```python
from build123d import *

# Parameters (mm, degrees)
F0_R     = 76.2
F0_W     = 60.587234
F0_H     = 3.302
F1_DEPTH = 12.7


with BuildPart() as f1:
    # F0 (on Front) → F1 (new body)
    with BuildSketch(Plane.XZ):
        Circle(F0_R)
        with Locations((37.913617, -11.811)):
            Rectangle(F0_W, F0_H, mode=Mode.SUBTRACT)
        with BuildLine():
            ThreePointArc((0, -6.35), (-6.35, 0), (0, 6.35))
            Line((0, 6.35), (0, 10.16))
            Line((0, 10.16), (7.62, 10.16))
            Line((7.62, 10.16), (7.62, 1.651))
            Line((7.62, 1.651), (68.58, 1.651))
            Line((68.58, 1.651), (68.58, -1.651))
            Line((68.58, -1.651), (7.62, -1.651))
            Line((7.62, -1.651), (7.62, -10.16))
            Line((7.62, -10.16), (0, -10.16))
            Line((0, -10.16), (0, -6.35))
        make_face(mode=Mode.SUBTRACT)
        with Locations((37.913617, 11.811)):
            Rectangle(F0_W, F0_H, mode=Mode.SUBTRACT)
        with BuildLine():
            ThreePointArc((0, 6.35), (4.490128, 4.490128), (6.35, 0))
            Line((6.35, 0), (7.62, 0))
            Line((7.62, 0), (7.62, 1.651))
            Line((7.62, 1.651), (7.62, 10.16))
            Line((7.62, 10.16), (0, 10.16))
            Line((0, 10.16), (0, 6.35))
        make_face()
        with BuildLine():
            Line((7.62, 0), (6.35, 0))
            ThreePointArc((6.35, 0), (4.490128, -4.490128), (0, -6.35))
            Line((0, -6.35), (0, -10.16))
            Line((0, -10.16), (7.62, -10.16))
            Line((7.62, -10.16), (7.62, -1.651))
            Line((7.62, -1.651), (7.62, 0))
        make_face()
        Polygon((7.62, 1.651), (7.62, 0), (7.62, -1.651), (68.58, -1.651), (68.58, 1.651), align=None)
    extrude(amount=F1_DEPTH)


solid = f1.part
```
Part model, mm, in its own coordinate system. A direction names the side the tool comes from. Coordinates: 2 decimals unless noted, no trailing zeros. Order: outer loops, then holes, each group sorted by start corner. A loop starts at its lowest first (then second) coordinate and runs counter-clockwise, first axis right, second up. Notation, with made-up numbers: (-1, 11) -> (27, 11) arc R15 ccw to (27, 27) -> close; hole circle Ø6 at (-26, 88.25). An arc over 180 degrees is marked (long way). Put each result on its own line as item: value. Start each with the question number.
(1) Which spindle directions (+Z, -Z, +X, -X, +Y, -Y) get a long thin tool onto all of the face, cutting with end or side? Do faces 4 (the face through (16, -12.7, 1)), 5 (the face through (68.207, -6, -12)). Say none if no direction does.
(2) Mould opens along Z. For faces 1 (the face through (-60.47, -6.261, -46.367)), 2 (the face through (68.207, -6, 12)), 3 (the face through (16, 0, 1)) say: pulls with the +Z half, pulls with the -Z half, needs draft (parallel to the pull), parting line crosses it, or undercut.
(3) Band-saw the part on A-A (y = -6.5). Give the cut face in (x, z), then the cut area to 3 significant figures.
(4) Pin check, flat tips, straight feed: pin 1 Ø1.7 at (y, z) = (-6, -12) entering from +X; pin 2 Ø4 at (x, y) = (52, -6.5) entering from -Z; pin 3 Ø3 at (x, y) = (2, -11) entering from -Z; pin 4 Ø1 at (x, z) = (3, -36.5) entering from +Y. Stop position of each tip, or through.
(5) Band-saw the part on C-C (z = -54). Give the cut face in (x, y).
(6) Band-saw the part on D-D (x = -47.5). Give the cut face in (y, z), then the cut area to 3 significant figures.
(7) Band-saw the part on B-B (x = 62.5). Give the cut face in (y, z), then the cut area to 3 significant figures.
(8) Probe line 1 along Z through (x, y) = (61, -11.5); line 2 along Z through (x, y) = (36, -1); line 3 along X through (y, z) = (-5, 2). List the from-to ranges inside material, lowest first. Write a range as [from, to].
Determined:
1. face 4: +Z, -Z, +X, -X, -Y
1. face 5: +Y, -Y
2. face 1: parting line crosses it
2. face 2: undercut
2. face 3: needs draft
3. outline: circle Ø152.4 at (0, 0); hole circle Ø12.7 at (0, 0); hole (7.62, -13.46) -> (68.21, -13.46) -> (68.21, -10.16) -> (7.62, -10.16) -> close; hole (7.62, 10.16) -> (68.21, 10.16) -> (68.21, 13.46) -> (7.62, 13.46) -> close
3. area: 17,700 mm²
4. pin 1: stops at x = 75.38
4. pin 2: stops at z = -57.5
4. pin 3: stops at z = -76.2
4. pin 4: stops at y = 0
5. outline: (-53.76, -12.7) -> (53.76, -12.7) -> (53.76, 0) -> (-53.76, 0) -> close
6. outline: (-12.7, -59.58) -> (0, -59.58) -> (0, 59.58) -> (-12.7, 59.58) -> close
6. area: 1,510 mm²
7. outline: (-12.7, -43.59) -> (0, -43.59) -> (0, -13.46) -> (-12.7, -13.46) -> close; (-12.7, -10.16) -> (0, -10.16) -> (0, 10.16) -> (-12.7, 10.16) -> close; (-12.7, 13.46) -> (0, 13.46) -> (0, 43.59) -> (-12.7, 43.59) -> close
7. area: 1,020 mm²
8. line 1: z = [-45.67, -13.46], [-10.16, 10.16], [13.46, 45.67]
8. line 2: z = [-67.16, -13.46], [-10.16, 10.16], [13.46, 67.16]
8. line 3: x = [-76.17, -6.03], [6.03, 76.17]
